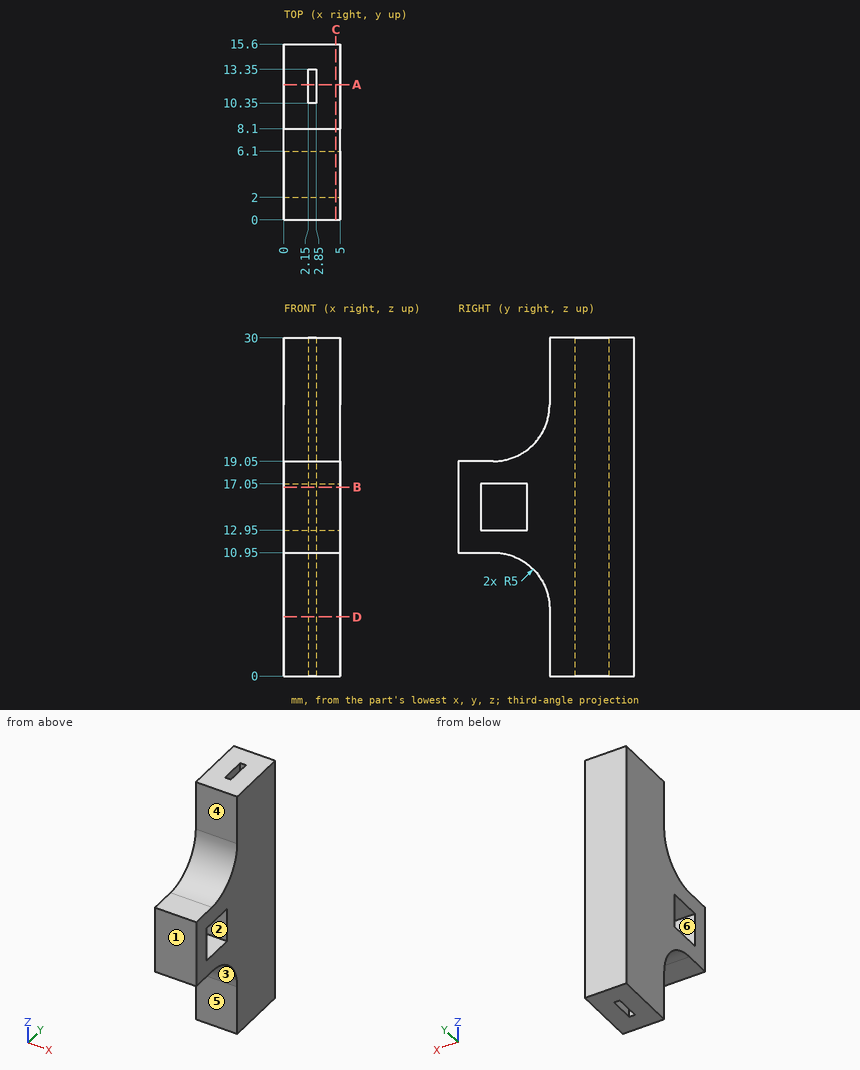
Could you check a few things on this drawing? It's one solid part, dimensions in mm from its lowest x, y, z. A direction names the side the tool comes from. Round coordinates to 2 decimals unless told otherwise and drop trailing zeros. Write each loop counter-clockwise with the first axis right and the second up, starting at its lowest first coordinate (ties: lowest second). Pieces come first, ordered by that corner, then holes. Notation, with made-up numbers: (22.5, 83) -> (46.5, 83) arc R16 cw to (46.5, 103) -> close; hole circle Ø8 at (6.25, -27). An arc over 180 degrees is marked (long way). Use a Markdown table: item, result.
1. Which directions (+Z, -Z, +X, -X, +Y, -Y) give clear straight access to the entire face, cutting with the end or side of a thin tool? Please do the marked faces 4, 5 and 6.
Answer key:
| item | result |
|---|---|
| face 4 | +Z, +X, -X, -Y |
| face 5 | -Z, +X, -X, -Y |
| face 6 | +X, -X |
2. If we section it at C-C (x = 4.6): List the corners of the cut face in (y, z) for me.
Answer key:
| item | result |
|---|---|
| outline | (0, 10.95) -> (3.1, 10.95) arc R5 cw to (8.1, 5.95) -> (8.1, 0) -> (15.6, 0) -> (15.6, 30) -> (8.1, 30) -> (8.1, 24.05) arc R5 cw to (3.1, 19.05) -> (0, 19.05) -> close; hole (2, 12.95) -> (6.1, 12.95) -> (6.1, 17.05) -> (2, 17.05) -> close |
3. For pin 1 Ø1 at (x, y) = (3, 3) entering from +Z; pin 2 Ø1 at (x, z) = (1, 21) entering from -Y; pin 3 Ø3 at (x, y) = (1.5, 5.5) entering from +Z, each with a flat end and sliding along its axis, tell me the tip position at first contact or that it passes through.
Answer key:
| item | result |
|---|---|
| pin 1 | stops at z = 19.07 |
| pin 2 | stops at y = 6.62 |
| pin 3 | stops at z = 20.92 |
4. If we section it at A-A (y = 12): List the corners of the cut face in (x, z) for me.
Answer key:
| item | result |
|---|---|
| outline | (0, 0) -> (2.15, 0) -> (2.15, 30) -> (0, 30) -> close; (2.85, 0) -> (5, 0) -> (5, 30) -> (2.85, 30) -> close |
5. If we section it at D-D (z = 5.25): List the corners of the cut face in (x, y) for me.
Answer key:
| item | result |
|---|---|
| outline | (0, 8.1) -> (5, 8.1) -> (5, 15.6) -> (0, 15.6) -> close; hole (2.15, 10.35) -> (2.85, 10.35) -> (2.85, 13.35) -> (2.15, 13.35) -> close |
6. We'd pull the mould along Z, two halves only. Please class the marked faces 1, 2 and 3: +Z half, -Z half, draft (parallel to the pull), parting line (faces both ways), or undercut.
Answer key:
| item | result |
|---|---|
| face 1 | draft |
| face 2 | undercut |
| face 3 | -Z half |
7. Please list where these lines run through material, in increasing order: probe 1 along Y at (x, z) = (4.3, 16.75); probe 2 along Z at (x, y) = (0.9, 2.25); probe 3 along X at (y, z) = (12.5, 12.5).
Answer key:
| item | result |
|---|---|
| probe 1 | y = 0 to 2, 6.1 to 15.6 |
| probe 2 | z = 10.95 to 12.95, 17.05 to 19.05 |
| probe 3 | x = 0 to 2.15, 2.85 to 5 |
8. If we section it at B-B (z = 16.75): List the corners of the cut face in (x, y) for me.
Answer key:
| item | result |
|---|---|
| outline | (0, 0) -> (5, 0) -> (5, 2) -> (0, 2) -> close; (0, 6.1) -> (5, 6.1) -> (5, 15.6) -> (0, 15.6) -> close; hole (2.15, 10.35) -> (2.85, 10.35) -> (2.85, 13.35) -> (2.15, 13.35) -> close |
